Source: CAD feature listing. Evaluate the final solid. Frame: model axes, mm. Face numbers are marked on the shaded views. A direction names the side the tool comes from. Give positions to 0.01 mm unless a question says otherwise; leave off trailing zeros. Loops run counter-clockwise (first coordinate to the right, second up) from the corner with the lowest first, then second, coordinate; pieces in that order, holes last.
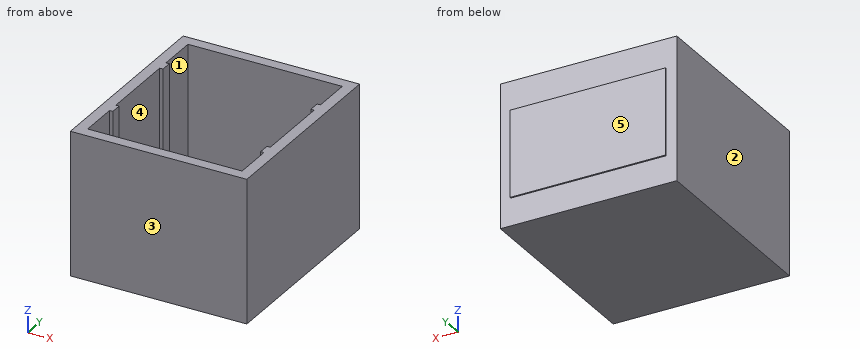
from build123d import *

# Parameters (mm, degrees)
SKETCH1_W           = 406.4
SKETCH1_H           = 457.2
BOSS_EXTRUDE1_DEPTH = 330.2
SHELL1_T            = -25.4
SKETCH2_W           = 304.8
SKETCH2_H           = 25.4
BOSS_EXTRUDE2_DEPTH = 7.62
SCALE1_SCALE        = 0.75
SKETCH3_W           = 267.97
SKETCH3_H           = 149.225
BOSS_EXTRUDE3_DEPTH = 2.54


with BuildPart() as part:
    # Sketch1 → Boss-Extrude1 (new body)
    with BuildSketch(Plane.XY):
        Rectangle(SKETCH1_W, SKETCH1_H)
    extrude(amount=-BOSS_EXTRUDE1_DEPTH)

    # Shell1
    shell1_openings = [part.faces().sort_by_distance(p)[0] for p in [
        (0, 0, 0),
    ]]
    offset(amount=SHELL1_T, openings=shell1_openings, kind=Kind.INTERSECTION)

    # Sketch2 → Boss-Extrude2 (add)
    with BuildSketch(Plane(origin=(-177.8, 0, 0), x_dir=(0, 0, -1), z_dir=(1, 0, 0))):
        with Locations((152.4, -101.6)):
            Rectangle(SKETCH2_W, SKETCH2_H)
        with Locations((152.4, 101.6)):
            Rectangle(SKETCH2_W, SKETCH2_H)
    boss_extrude2 = extrude(amount=BOSS_EXTRUDE2_DEPTH)

    # Mirror1: Boss-Extrude2 across plane
    add(boss_extrude2.mirror(Plane(origin=(0, 0, 0), x_dir=(0, 0, 1), z_dir=(1, 0, 0))))


with BuildPart() as part_1:
    # Scale1: scaled about (0, 0, -196.821524664)
    add(part.part.scale(SCALE1_SCALE).moved(Location((0, 0, -49.205381166))))

    # Sketch3 → Boss-Extrude3 (add)
    with BuildSketch(Plane(origin=(0, 171.45, 0), x_dir=(1, 0, 0), z_dir=(0, 1, 0))):
        with Locations((0, 174.617881166)):
            Rectangle(SKETCH3_W, SKETCH3_H)
    extrude(amount=BOSS_EXTRUDE3_DEPTH)


solid = part_1.part
1) Ray query, probe 1 along Y at (x, z) = (-115, -197.5); probe 2 along X at (y, z) = (-40.5, -153); probe 3 along Y at (x, z) = (128, -183) (3 decimals). Return the intervals inside material, ascending.
Checks:
probe 1: y = -171.45 to -152.4, 152.4 to 173.99
probe 2: x = -152.4 to -133.35, 133.35 to 152.4
probe 3: y = -171.45 to -152.4, -85.725 to -66.675, 66.675 to 85.725, 152.4 to 173.99
2) Cut plane D-D (z = -65.5). Return loops of the section in (x, y) (3 decimals).
Checks:
outline: (-152.4, -171.45) - (152.4, -171.45) - (152.4, 171.45) - (-152.4, 171.45) - close; hole (-133.35, -152.4) - (133.35, -152.4) - (133.35, -85.725) - (127.635, -85.725) - (127.635, -66.675) - (133.35, -66.675) - (133.35, 66.675) - (127.635, 66.675) - (127.635, 85.725) - (133.35, 85.725) - (133.35, 152.4) - (-133.35, 152.4) - (-133.35, 85.725) - (-127.635, 85.725) - (-127.635, 66.675) - (-133.35, 66.675) - (-133.35, -66.675) - (-127.635, -66.675) - (-127.635, -85.725) - (-133.35, -85.725) - close
3) Cut plane C-C (x = 85). Return loops of the section in (y, z), and give its area (3 significant figures).
Checks:
outline: (-171.45, -296.86) - (171.45, -296.86) - (171.45, -249.23) - (173.99, -249.23) - (173.99, -100.01) - (171.45, -100.01) - (171.45, -49.21) - (152.4, -49.21) - (152.4, -277.81) - (-152.4, -277.81) - (-152.4, -49.21) - (-171.45, -49.21) - close
area: 15,600 mm2
4) Contact query for flat-ended pins moving along their axis: P1, Ø10, axis at x = -54, y = 70, coming from the +Z side; P2, Ø2, axis at y = 172.5, z = -159, coming from the +X side (3 decimals). Output: stop coordinate, or through.
Checks:
P1: stops at z = -277.81
P2: stops at x = 133.985
5) Cut plane B-B (y = 80). Return loops of the section in (x, z) (3 decimals).
Checks:
outline: (-152.4, -296.855) - (152.4, -296.855) - (152.4, -49.205) - (127.635, -49.205) - (127.635, -277.805) - (-127.635, -277.805) - (-127.635, -49.205) - (-152.4, -49.205) - close
6) Pull-direction query (X, two-part tool) for the marked faces 1, 2 and 3; classes: released by +X, released by -X, zero draft, split by the parting line, or undercut.
Checks:
face 1: undercut
face 2: released by -X
face 3: zero draft
7) Reachability of the marked faces 4 and 5 from +Z, -Z, +X, -X, +Y, -Y: full face, straight path, thin tool, end or side. Return the list, or none.
Checks:
face 4: +Z
face 5: +Z, -Z, +X, -X, +Y
8) Cut plane A-A (z = -159.5). Return loops of the section in (x, y) (3 decimals), and give its area (3 significant figures).
Checks:
outline: (-152.4, -171.45) - (152.4, -171.45) - (152.4, 171.45) - (133.985, 171.45) - (133.985, 173.99) - (-133.985, 173.99) - (-133.985, 171.45) - (-152.4, 171.45) - close; hole (-133.35, -152.4) - (133.35, -152.4) - (133.35, -85.725) - (127.635, -85.725) - (127.635, -66.675) - (133.35, -66.675) - (133.35, 66.675) - (127.635, 66.675) - (127.635, 85.725) - (133.35, 85.725) - (133.35, 152.4) - (-133.35, 152.4) - (-133.35, 85.725) - (-127.635, 85.725) - (-127.635, 66.675) - (-133.35, 66.675) - (-133.35, -66.675) - (-127.635, -66.675) - (-127.635, -85.725) - (-133.35, -85.725) - close
area: 24,300 mm2
